Source: CAD feature listing. Evaluate the final solid. Frame: model axes, mm. A direction names the side the tool comes from. Give positions to 0.01 mm unless a question says otherwise; leave off trailing zeros. Loops run counter-clockwise (first coordinate to the right, second up) from the corner with the lowest first, then second, coordinate; pieces in that order, holes last. Notation, with made-up numbers: M 53,31.5 L 112,31.5 A13 ccw 112,35.5 Z; hole C 73,16 d9. An arc over 180 degrees is marked long. Put each result on its own line as item: value.
from build123d import *

# Parameters (mm, degrees)
SKETCH1_W           = 70
SKETCH1_H           = 70
SKETCH1_R           = 31
BOSS_EXTRUDE1_DEPTH = 15
SKETCH2_R           = 2.5
CUT_EXTRUDE1_DEPTH  = 52.720402164
FILLET1_R           = 5
SKETCH3_R           = 5
CUT_EXTRUDE2_DEPTH  = 3


with BuildPart() as part:
    # Sketch1 → Boss-Extrude1 (new body)
    with BuildSketch(Plane(origin=(0, 0, 0), x_dir=(1, 0, 0), z_dir=(0, 1, 0))):
        Rectangle(SKETCH1_W, SKETCH1_H)
        with Locations(Location((0, 0, 0), (0, 0, 270))):
            Circle(SKETCH1_R, mode=Mode.SUBTRACT)
    extrude(amount=BOSS_EXTRUDE1_DEPTH)

    # Sketch2 → Cut-Extrude1 (cut, through all)
    with BuildSketch(Plane(origin=(0, 15, 0), x_dir=(1, 0, 0), z_dir=(0, 1, 0))):
        with Locations(Location((-28, 28, 0), (0, 0, 270))):
            Circle(SKETCH2_R)
        with Locations(Location((28, 28, 0), (0, 0, 90))):
            Circle(SKETCH2_R)
        with Locations(Location((28, -28, 0), (0, 0, 270))):
            Circle(SKETCH2_R)
        with Locations(Location((-28, -28, 0), (0, 0, 90))):
            Circle(SKETCH2_R)
    extrude(amount=-CUT_EXTRUDE1_DEPTH, mode=Mode.SUBTRACT)

    # Fillet1
    fillet1_edges = [part.edges().sort_by_distance(p)[0] for p in [
        (35, 7.5, 35),
        (-35, 7.5, 35),
        (-35, 7.5, -35),
        (35, 7.5, -35),
    ]]
    fillet(fillet1_edges, radius=FILLET1_R)

    # Sketch3 → Cut-Extrude2 (cut)
    with BuildSketch(Plane(origin=(0, 15, 0), x_dir=(1, 0, 0), z_dir=(0, 1, 0))):
        with Locations(Location((-28, 28, 0), (0, 0, 270))):
            Circle(SKETCH3_R)
        with Locations(Location((-28, -28, 0), (0, 0, 90))):
            Circle(SKETCH3_R)
        with Locations(Location((28, 28, 0), (0, 0, 90))):
            Circle(SKETCH3_R)
        with Locations(Location((28, -28, 0), (0, 0, 270))):
            Circle(SKETCH3_R)
    extrude(amount=-CUT_EXTRUDE2_DEPTH, mode=Mode.SUBTRACT)


solid = part.part
1. Section query C-C (x = 0). Output: boundary loops of the cut face in (y, z), plus the area to 3 significant figures.
Found:
outline: M 0,-35 L 15,-35 L 15,-31 L 0,-31 Z; M 0,31 L 15,31 L 15,35 L 0,35 Z
area: 120 mm^2
2. Access query for faces 1 (the cylindrical face through (-25, 14, 32)), 2 (the cylindrical face through (30.48, 6.08, 27.67)). Directions: +Z, -Z, +X, -X, +Y, -Y. A direction counts if a zero-diameter tool reaches every point of the face in a straight line with its end or side. Return the directions, or none.
Found:
face 1: +Y
face 2: +Y, -Y
3. Contact query for flat-ended pins moving along their axis: P1, Ø8, axis at x = 28, z = -28, coming from the -Y side; P2, Ø3, axis at x = 29, z = -29, coming from the +Y side. Output: stop coordinate, or through.
Found:
P1: y = 0
P2: y = 12
4. Draft query along X for faces 3 (the flat face through (35, 7, 0)), 4 (the flat face through (-13.1, 15, 28.4)), 5 (the cylindrical face through (31, 14, -24)). Return one class per face: pulls with the +X half, pulls with the -X half, needs draft (parallel to the pull), parting line crosses it, or undercut.
Found:
face 3: pulls with the +X half
face 4: needs draft
face 5: undercut
5. Material intervals for line 1 (X direction, y = 3, z = -28); line 2 (X direction, y = 13.8, z = -28); line 3 (Z direction, x = 28.5, y = 10.25), sorted ascending. Write a range as from..to.
Found:
line 1: -35..-30.5, -25.5..-13.3, 13.3..25.5, 30.5..35
line 2: -35..-33, -23..-13.3, 13.3..23, 33..35
line 3: -35..-30.45, -25.55..-12.2, 12.2..25.55, 30.45..35
6. Section query B-B (y = 7.5). Output: boundary loops of the cut face in (x, z).
Found:
outline: M -35,-30 A5 ccw -30,-35 L 30,-35 A5 ccw 35,-30 L 35,30 A5 ccw 30,35 L -30,35 A5 ccw -35,30 Z; hole C 0,0 d62; hole C -28,-28 d5; hole C -28,28 d5; hole C 28,-28 d5; hole C 28,28 d5
7. Section query D-D (x = 28). Output: boundary loops of the cut face in (y, z), plus the area to 3 significant figures.
Found:
outline: M 0,-35 L 15,-35 L 15,-33 L 12,-33 L 12,-30.5 L 0,-30.5 Z; M 0,-25.5 L 12,-25.5 L 12,-23 L 15,-23 L 15,-13.3 L 0,-13.3 Z; M 0,13.3 L 15,13.3 L 15,23 L 12,23 L 12,25.5 L 0,25.5 Z; M 0,30.5 L 12,30.5 L 12,33 L 15,33 L 15,35 L 0,35 Z
area: 471 mm^2
8. Section query A-A (z = 0). Output: boundary loops of the cut face in (x, y), plus the area to 3 significant figures.
Found:
outline: M -35,0 L -31,0 L -31,15 L -35,15 Z; M 31,0 L 35,0 L 35,15 L 31,15 Z
area: 120 mm^2
